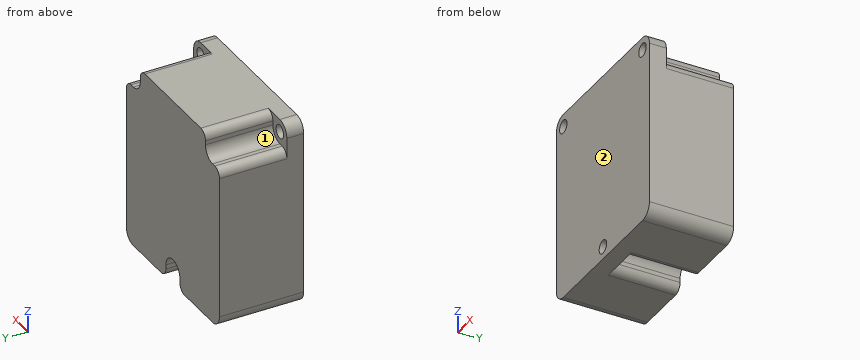
from build123d import *

# Parameters (mm, degrees)
SKETCH_1_R          = 1.6
EXTRUDE_1_DEPTH     = 20
SKETCH_2_R          = 1.6
CUT_EXTRUDE_1_DEPTH = 16
FILLET_1_R          = 2
SKETCH_3_R          = 7
EXTRUDE_2_DEPTH     = 50
SKETCH_4_R          = 7
CUT_EXTRUDE_2_DEPTH = 50


with BuildPart() as part:
    # 草图1 → 凸台-拉伸1 (new body)
    with BuildSketch(Plane(origin=(0, 0, 0), x_dir=(1, 0, 0), z_dir=(0, 1, 0))):
        with BuildLine():
            Line((3, 0), (37, 0))
            ThreePointArc((37, 0), (39.121320344, -0.878679656), (40, -3))
            Line((40, -3), (40, -42))
            ThreePointArc((40, -42), (39.121320344, -44.121320344), (37, -45))
            Line((37, -45), (3, -45))
            ThreePointArc((3, -45), (0.878679656, -44.121320344), (0, -42))
            Line((0, -42), (0, -3))
            ThreePointArc((0, -3), (0.878679656, -0.878679656), (3, 0))
        make_face()
        with Locations((20, -3)):
            Circle(SKETCH_1_R, mode=Mode.SUBTRACT)
        with Locations((3, -42)):
            Circle(SKETCH_1_R, mode=Mode.SUBTRACT)
        with Locations((37, -42)):
            Circle(SKETCH_1_R, mode=Mode.SUBTRACT)
    extrude(amount=EXTRUDE_1_DEPTH)

    # 草图2 → 切除-拉伸1 (cut)
    with BuildSketch(Plane(origin=(0, 20, 0), x_dir=(1, 0, 0), z_dir=(0, 1, 0))):
        with BuildLine():
            Line((40, -42), (40, -39))
            Line((40, -39), (37, -39))
            ThreePointArc((37, -39), (34.878679656, -39.878679656), (34, -42))
            Line((34, -42), (34, -45))
            Line((34, -45), (37, -45))
            ThreePointArc((37, -45), (39.121320344, -44.121320344), (40, -42))
        make_face()
        with Locations((37, -42)):
            Circle(SKETCH_2_R, mode=Mode.SUBTRACT)
        with BuildLine():
            Line((3, -39), (0, -39))
            Line((0, -39), (0, -42))
            ThreePointArc((0, -42), (0.878679656, -44.121320344), (3, -45))
            Line((3, -45), (6, -45))
            Line((6, -45), (6, -42))
            ThreePointArc((6, -42), (5.121320344, -39.878679656), (3, -39))
        make_face()
        with Locations((3, -42)):
            Circle(SKETCH_2_R, mode=Mode.SUBTRACT)
        with BuildLine():
            Line((17, 0), (17, -3))
            ThreePointArc((17, -3), (20, -6), (23, -3))
            Line((23, -3), (23, 0))
            Line((23, 0), (17, 0))
        make_face()
        with Locations((20, -3)):
            Circle(SKETCH_2_R, mode=Mode.SUBTRACT)
    extrude(amount=-CUT_EXTRUDE_1_DEPTH, mode=Mode.SUBTRACT)

    # 圆角1
    fillet_1_edges = [part.edges().sort_by_distance(p)[0] for p in [
        (40, 12, 39),
        (34, 12, 45),
        (6, 12, 45),
        (0, 12, 39),
        (17, 12, 0),
        (23, 12, 0),
    ]]
    fillet(fillet_1_edges, radius=FILLET_1_R)

    # 草图3 → 凸台-拉伸2 (add)
    with BuildSketch(Plane.XY.offset(45)):
        with Locations((20, 10)):
            Circle(SKETCH_3_R)
    extrude(amount=EXTRUDE_2_DEPTH)

    # 草图4 → 切除-拉伸2 (cut)
    with BuildSketch(Plane.XY.offset(95)):
        with Locations((20, 10)):
            Circle(SKETCH_4_R)
    extrude(amount=-CUT_EXTRUDE_2_DEPTH, mode=Mode.SUBTRACT)


solid = part.part
Geometry check sheet. Reference: the model listing, model coordinates, mm. Face numbers are marked on the shaded views. A direction names the side the tool comes from. Round coordinates to 2 decimals unless told otherwise and drop trailing zeros. Order: outer loops, then holes, each group sorted by start corner. A loop starts at its lowest first (then second) coordinate and runs counter-clockwise, first axis right, second up. Notation, with made-up numbers: (24, 25) -> (39, 25) arc R14 cw to (39, 40) -> close; hole circle Ø3 at (-33.75, -15.75). An arc over 180 degrees is marked (long way). Use one line per item in the form item = value.
1. Cross-section at B-B, the plane z = 4. Enter the section's corners in (x, y).
Working result:
outline = (0, 0) -> (18.75, 0) -> (18.75, 4) -> (17.17, 4) -> (17.17, 20) -> (0, 20) -> close; (21.25, 0) -> (40, 0) -> (40, 20) -> (22.83, 20) -> (22.83, 4) -> (21.25, 4) -> close
2. Scan lines: line 1 along X through (y, z) = (3.1, 42); line 2 along Z through (x, y) = (37, 0.95); line 3 along Z through (x, y) = (20, 2.7). Record each from-to range of solid material in increasing order. Write a range as from..to.
Working result:
line_1 = 0..1.4, 4.6..35.4, 38.6..40
line_2 = 0..40.4, 43.6..45
line_3 = 0..1.4, 4.6..45
3. Cross-section at A-A, the plane x = 20. Enter the section's corners in (y, z).
Working result:
outline = (0, 0) -> (4, 0) -> (4, 1.4) -> (0, 1.4) -> close; (0, 4.6) -> (4, 4.6) -> (4, 6) -> (20, 6) -> (20, 45) -> (0, 45) -> close
4. Go/stop test with flat-tipped pins: pin 1 (5 mm diameter, centred on x = 19.5, z = 20.5, fed in from -Y); pin 2 (2.5 mm diameter, centred on x = 37.5, z = 42.5, fed in from +Y); pin 3 (0.8 mm diameter, centred on x = 37.5, y = 10, fed in from +Z); pin 4 (0.5 mm diameter, centred on y = 8, z = 2.5, fed in from -X). Record where each tip stops, or that it passes through.
Working result:
pin_1 = 0
pin_2 = 4
pin_3 = 39
pin_4 = 0.01
5. Set-up check for the marked faces 1 and 2: record each of +Z, -Z, +X, -X, +Y, -Y from which the full face is reachable in a straight line by a thin tool's end or side.
Working result:
face_1 = +Z, -X, +Y
face_2 = +Z, -Z, +X, -X, -Y
